Here's how the part is built. I have some questions about the finished solid (model axes, mm). Face numbers are marked on the shaded views. A direction names the side the tool comes from. Coordinates: 2 decimals unless noted, no trailing zeros. Write each loop counter-clockwise with the first axis right and the second up, starting at its lowest first coordinate (ties: lowest second). Pieces come first, ordered by that corner, then holes.
```python
from build123d import *

# Parameters (mm, degrees)
RESSALTO_EXTRUS_O1_DEPTH   = 10
ESBO_O2_R                  = 2
CORTE_EXTRUS_O1_DEPTH      = 8
CORTE_EXTRUS_O2_DEPTH      = 61.737138556
CORTE_EXTRUS_O2_DEPTH_BACK = 61.737138556
ESBO_O3_R                  = 1.15


with BuildPart() as part:
    # Esboço1 → Ressalto-extrusão1 (new, symmetric)
    with BuildSketch(Plane.XY):
        Polygon((0, 0), (0, 10), (-58, 10), (-58, 15), (6, 15), (6, 0), align=None)
    extrude(amount=RESSALTO_EXTRUS_O1_DEPTH, both=True)

    # Esboço2 → Corte-extrusão1 (cut)
    with BuildSketch(Plane.ZY):
        with Locations(Location((-4, 5, 0), (0, 0, 270))):
            Circle(ESBO_O2_R)
        with Locations(Location((4, 5, 0), (0, 0, 270))):
            Circle(ESBO_O2_R)
    extrude(amount=-CORTE_EXTRUS_O1_DEPTH, mode=Mode.SUBTRACT)

    # Esboço3 → Corte-extrusão2 (cut, two sides: drawn at the far end of the back side and taken through both)
    with BuildSketch(Plane(origin=(0, 15, 0), x_dir=(1, 0, 0), z_dir=(0, 1, 0)).offset(-CORTE_EXTRUS_O2_DEPTH_BACK)):
        with Locations(Location((-16, -7.65, 0), (0, 0, 180))):
            Circle(ESBO_O3_R)
        with Locations(Location((-22.4, -7.65, 0), (0, 0, 180))):
            Circle(ESBO_O3_R)
        with Locations(Location((-35.5, -7.65, 0), (0, 0, 180))):
            Circle(ESBO_O3_R)
        with Locations(Location((-41.9, -7.65, 0), (0, 0, 180))):
            Circle(ESBO_O3_R)
        with Locations(Location((-46, 7.65, 0), (0, 0, 180))):
            Circle(ESBO_O3_R)
        with Locations(Location((-52.4, 7.65, 0), (0, 0, 180))):
            Circle(ESBO_O3_R)
        with Locations(Location((-13.4, 7.65, 0), (0, 0, 180))):
            Circle(ESBO_O3_R)
        with Locations(Location((-7, 7.65, 0), (0, 0, 180))):
            Circle(ESBO_O3_R)
    extrude(amount=CORTE_EXTRUS_O2_DEPTH + CORTE_EXTRUS_O2_DEPTH_BACK, mode=Mode.SUBTRACT)


solid = part.part
```
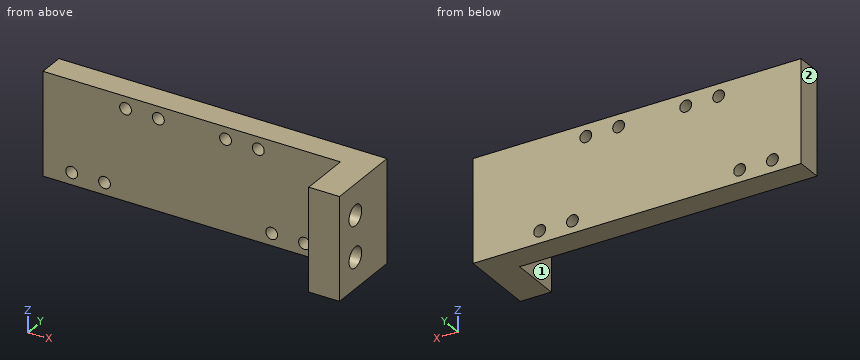
1) I need wall thicknesses on probe 1 along X at (y, z) = (13.3, 7.65); probe 2 along Z at (x, y) = (-46, 13.1); probe 3 along X at (y, z) = (14, -7). Which ranges of each line are inside material? Lowest first, please.
Values follow:
probe 1: x = -58 to -43.05, -40.75 to -36.65, -34.35 to -23.55, -21.25 to -17.15, -14.85 to 6
probe 2: z = -10 to -8.8, -6.5 to 10
probe 3: x = -58 to -53.35, -51.45 to -46.95, -45.05 to -14.35, -12.45 to -7.95, -6.05 to 6
2) Imagine slicing it at D-D on x = -32. Please give me the cut outline in (y, z).
Values follow:
outline: (10, -10) - (15, -10) - (15, 10) - (10, 10) - close
3) Imagine slicing it at A-A on x = -46. Please give me the cut outline in (y, z).
Values follow:
outline: (10, -10) - (15, -10) - (15, -8.8) - (10, -8.8) - close; (10, -6.5) - (15, -6.5) - (15, 10) - (10, 10) - close
4) Imagine slicing it at B-B on z = 7.65. Please give me the cut outline in (x, y).
Values follow:
outline: (-58, 10) - (-43.05, 10) - (-43.05, 15) - (-58, 15) - close; (-40.75, 10) - (-36.65, 10) - (-36.65, 15) - (-40.75, 15) - close; (-34.35, 10) - (-23.55, 10) - (-23.55, 15) - (-34.35, 15) - close; (-21.25, 10) - (-17.15, 10) - (-17.15, 15) - (-21.25, 15) - close; (-14.85, 10) - (0, 10) - (0, 0) - (6, 0) - (6, 15) - (-14.85, 15) - close
5) Will these pins go through, and if not, where does the flat tip stop? pin 1 (6 mm diameter, centred on y = 4.5, z = -2, fed in from -X); pin 2 (3 mm diameter, centred on x = -25, z = -1.5, fed in from -Y).
Values follow:
pin 1: stops at x = 0
pin 2: stops at y = 10
6) Imagine slicing it at C-C on y = 5.5. Please give me the cut outline in (x, z).
Values follow:
outline: (0, -10) - (6, -10) - (6, -5.94) - (0, -5.94) - close; (0, -2.06) - (6, -2.06) - (6, 2.06) - (0, 2.06) - close; (0, 5.94) - (6, 5.94) - (6, 10) - (0, 10) - close
7) On a 3-axis mill with a long thin cutter (end or side, diameter ignored), from which of +Z, -Z, +X, -X, +Y, -Y can I reach the whole of each face in a straight line? I mean the marked faces 1 and 2. Say none if no direction works.
Values follow:
face 1: +Z, -Z, -X, -Y
face 2: +Z, -Z, -X, +Y, -Y
